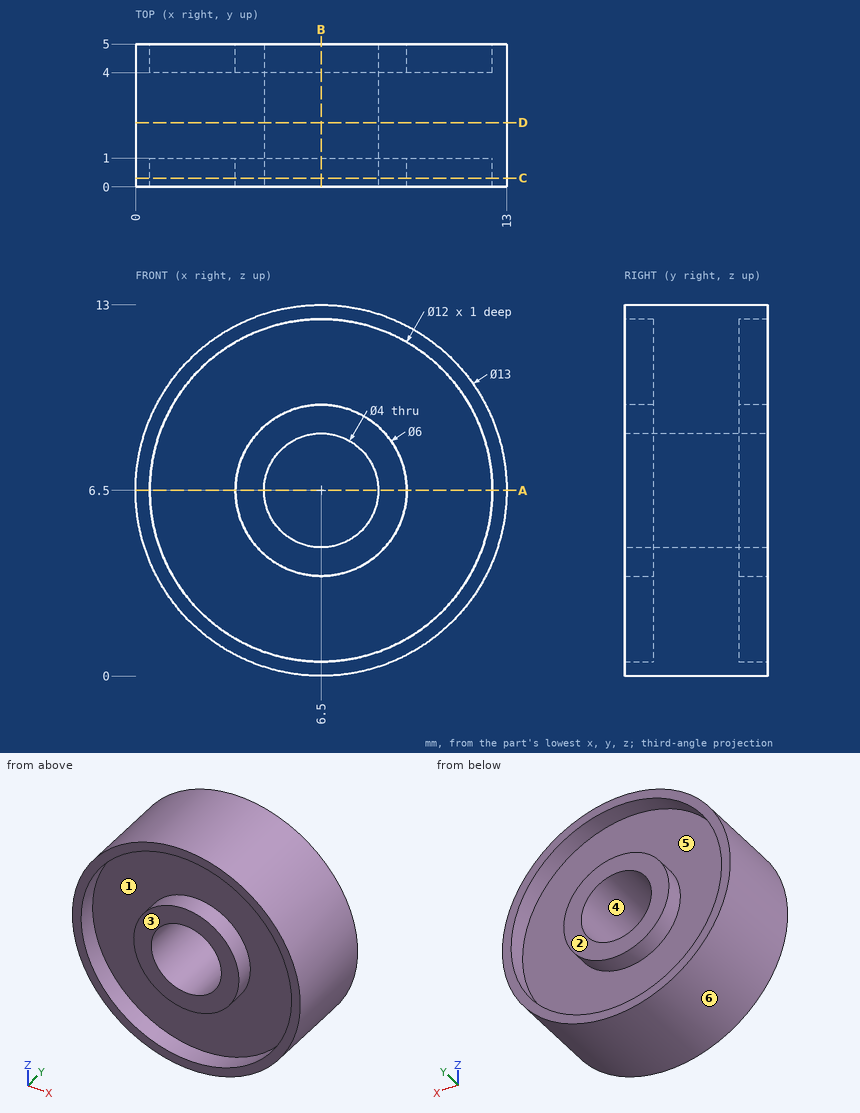
The drawing under review shows one solid part. Ordinate dimensions are in mm from its lowest x, y, z. A direction names the side the tool comes from. Give positions to 0.01 mm unless a question says otherwise; leave off trailing zeros. Write each loop counter-clockwise with the first axis right and the second up, starting at its lowest first coordinate (ties: lowest second). Pieces come first, ordered by that corner, then holes. Notation, with made-up numbers: (37, 33.5) -> (75, 33.5) arc R12 cw to (75, 53.5) -> close; hole circle Ø5 at (89, 32.25). An arc over 180 degrees is marked (long way). Use CSV: the item, a comma, the result in double quotes.
Q1. Take a section at A-A, the plane z = 6.5. Write out the cut boundary in (x, y), then the cut area to 3 significant figures.
Conclusion:
outline,"(0, 0) -> (0.5, 0) -> (0.5, 1) -> (3.5, 1) -> (3.5, 0) -> (4.5, 0) -> (4.5, 5) -> (3.5, 5) -> (3.5, 4) -> (0.5, 4) -> (0.5, 5) -> (0, 5) -> close; (8.5, 0) -> (9.5, 0) -> (9.5, 1) -> (12.5, 1) -> (12.5, 0) -> (13, 0) -> (13, 5) -> (12.5, 5) -> (12.5, 4) -> (9.5, 4) -> (9.5, 5) -> (8.5, 5) -> close"
area,"33.0 mm2"
Q2. Take a section at D-D, the plane y = 2.25. Write out the cut boundary in (x, z), then the cut area to 3 significant figures.
Conclusion:
outline,"circle Ø13 at (6.5, 6.5); hole circle Ø4 at (6.5, 6.5)"
area,"120 mm2"
Q3. For P1, Ø1, axis at x = 2, z = 9.5, coming from the -Y side; P2, Ø1, axis at x = 9.5, y = 4, coming from the +Z side; P3, Ø2, axis at x = 1.5, y = 1.5, coming from the -Z side; P4, Ø3, axis at x = 6.5, z = 6.5, coming from the +Y side, all flat-tipped, find the tip position at first contact; note any pin that passes through.
Conclusion:
P1,"y = 1"
P2,"z = 12.5"
P3,"z = 1.38"
P4,"through"
Q4. To check wall thickness, follow probe 1 along X at (y, z) = (0.2, 6.5); probe 2 along X at (y, z) = (2.05, 6.5); probe 3 along Z at (x, y) = (5, 4.65). State the ranges of each line that lie inside material, in increasing order. Write a range as [from, to].
Conclusion:
probe 1,"[0, 0.5], [3.5, 4.5], [8.5, 9.5], [12.5, 13]"
probe 2,"[0, 4.5], [8.5, 13]"
probe 3,"[0.18, 0.69], [3.9, 5.18], [7.82, 9.1], [12.31, 12.82]"
Q5. Take a section at C-C, the plane y = 0.3. Write out the cut boundary in (x, z).
Conclusion:
outline,"circle Ø13 at (6.5, 6.5); circle Ø6 at (6.5, 6.5); hole circle Ø12 at (6.5, 6.5); hole circle Ø4 at (6.5, 6.5)"
Q6. Tool access review of the marked faces 1 and 2: name each direction out of +Z, -Z, +X, -X, +Y, -Y from which nothing blocks a thin tool from reaching the whole face with its end or side.
Conclusion:
face 1,"-Y"
face 2,"+Z, -Z, +X, -X, +Y"
Q7. Take a section at B-B, the plane x = 6.5. Write out the cut boundary in (y, z), then the cut area to 3 significant figures.
Conclusion:
outline,"(0, 0) -> (5, 0) -> (5, 0.5) -> (4, 0.5) -> (4, 3.5) -> (5, 3.5) -> (5, 4.5) -> (0, 4.5) -> (0, 3.5) -> (1, 3.5) -> (1, 0.5) -> (0, 0.5) -> close; (0, 8.5) -> (5, 8.5) -> (5, 9.5) -> (4, 9.5) -> (4, 12.5) -> (5, 12.5) -> (5, 13) -> (0, 13) -> (0, 12.5) -> (1, 12.5) -> (1, 9.5) -> (0, 9.5) -> close"
area,"33.0 mm2"
Q8. Mouldability with a two-part tool opening along X and no side actions: class the marked faces 3, 4, 5 and 6 as pulls with the +X half, pulls with the -X half, needs draft (parallel to the pull), parting line crosses it, or undercut.
Conclusion:
face 3,"needs draft"
face 4,"undercut"
face 5,"undercut"
face 6,"parting line crosses it"
